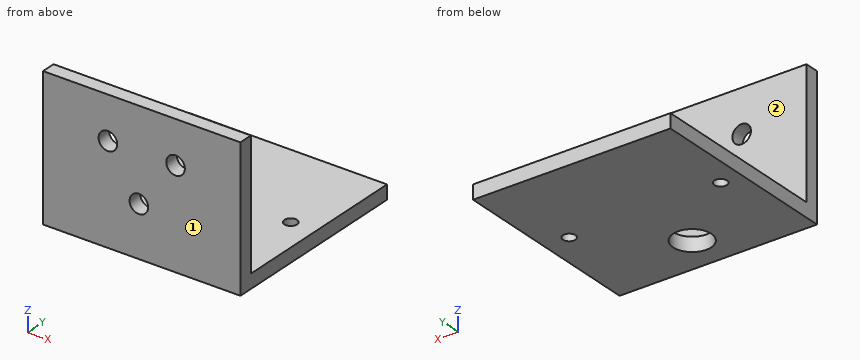
```python
from build123d import *

# Parameters (mm, degrees)
ESQUISSE1_W             = 70
ESQUISSE1_H             = 70
BOSS_EXTRU_1_DEPTH      = 50
ESQUISSE2_W             = 123.137615707
ESQUISSE2_H             = 86.86411441
ENL_V_MAT_EXTRU_1_DEPTH = 217
D_GAGEMENT_M41_D        = 4.5
D_GAGEMENT_M121_D       = 13.5
M6_CLEARANCE_HOLE1_D    = 6.6


with BuildPart() as part:
    # Esquisse1 → Boss.-Extru.1 (new body)
    with BuildSketch(Plane.XY):
        Rectangle(ESQUISSE1_W, ESQUISSE1_H)
    extrude(amount=BOSS_EXTRU_1_DEPTH)

    # Esquisse2 → Enlèv. mat.-Extru.1 (cut)
    with BuildSketch(Plane(origin=(35, 0, 0), x_dir=(0, 0, -1), z_dir=(1, 0, 0))):
        with Locations((-66.568807854, 13.432057205)):
            Rectangle(ESQUISSE2_W, ESQUISSE2_H)
    extrude(amount=-ENL_V_MAT_EXTRU_1_DEPTH, mode=Mode.SUBTRACT)

    # Dégagement M41 (through all)
    with Locations(Plane(origin=(0, 0, 0), x_dir=(-1, 0, 0), z_dir=(0, 0, -1))):
        with Locations((-26.157577905, 0.946358973), (27.533117647, 0.946358973)):
            Hole(D_GAGEMENT_M41_D / 2)

    # Dégagement M121 (through all)
    with Locations(Plane(origin=(0, 0, 0), x_dir=(-1, 0, 0), z_dir=(0, 0, -1))):
        with Locations((0.875458958, -21.366395267)):
            Hole(D_GAGEMENT_M121_D / 2)

    # M6 Clearance Hole1 (through all)
    with Locations(Plane(origin=(0, -30, 0), x_dir=(1, 0, 0), z_dir=(0, 1, 0))):
        with Locations((-12, -34.845648012), (12, -34.845648012), (-1, -18)):
            Hole(M6_CLEARANCE_HOLE1_D / 2)


solid = part.part
```
Model file for the job. Use its own axes, mm. Face numbers are marked on the shaded views. A direction names the side the tool comes from. Coordinates: 2 decimals unless noted, no trailing zeros. Write each loop counter-clockwise with the first axis right and the second up, starting at its lowest first coordinate (ties: lowest second). Pieces come first, ordered by that corner, then holes. Notation, with made-up numbers: (73.5, 55.25) - (103.5, 55.25) arc R27 cw to (103.5, 83.25) - close; hole circle Ø3 at (60.25, -15). An arc over 180 degrees is marked (long way). One line per item, written item: value. Start each with the question number.
1. Probe line 1 (Z direction, x = -12, y = -33); line 2 (Z direction, x = 8, y = -23.5); line 3 (Y direction, x = 3, z = 8). List the from-to ranges inside material, lowest first. Write a range as from..to.
2. Slice it at D-D (y = 14). Write the cut outline in (x, z).
3. Tool access for the marked faces 1 and 2: list every direction of +Z, -Z, +X, -X, +Y, -Y with a clear straight run to the whole face (end or side of a thin tool).
4. Flat gauge pins, fed straight in: pin 1 (13.5 mm diameter, centred on x = 12.5, z = 36, fed in from +Y); pin 2 (19.5 mm diameter, centred on x = -3, y = -11, fed in from +Z). Where does each tip first touch, or does it go through?
5. Slice it at A-A (x = 12). Write the cut outline in (y, z).
6. Slice it at B-B (x = -1). Write the cut outline in (y, z).
7. Slice it at C-C (z = 27). Write the cut outline in (x, y).
Answers below:
1. line 1: z = 0..31.55, 38.15..50
1. line 2: z = 0..5
1. line 3: y = -35..-30
2. outline: (-35, 0) - (35, 0) - (35, 5) - (-35, 5) - close
3. face 1: +Z, -Z, +X, -X, -Y
3. face 2: +Z, +X, -X, +Y
4. pin 1: stops at y = -30
4. pin 2: stops at z = 5
5. outline: (-35, 0) - (35, 0) - (35, 5) - (-30, 5) - (-30, 31.55) - (-35, 31.55) - close; (-35, 38.15) - (-30, 38.15) - (-30, 50) - (-35, 50) - close
6. outline: (-35, 0) - (-28.12, 0) - (-28.12, 5) - (-30, 5) - (-30, 14.7) - (-35, 14.7) - close; (-35, 21.3) - (-30, 21.3) - (-30, 50) - (-35, 50) - close; (-14.62, 0) - (35, 0) - (35, 5) - (-14.62, 5) - close
7. outline: (-35, -35) - (35, -35) - (35, -30) - (-35, -30) - close
